```python
from build123d import *

# Parameters (mm, degrees)
SKETCH1_W           = 80
SKETCH1_H           = 60
BOSS_EXTRUDE1_DEPTH = 10
BOSS_EXTRUDE2_DEPTH = 10
LPATTERN2_COUNT     = 2
LPATTERN2_PITCH     = 70
FILLET1_R           = 5
BOSS_EXTRUDE3_START = -33.53553
BOSS_EXTRUDE3_DEPTH = 5
SKETCH4_R           = 2
CUT_EXTRUDE1_DEPTH  = 11
CUT_EXTRUDE2_DEPTH  = 81


with BuildPart() as part:
    # Sketch1 → Boss-Extrude1 (new body)
    with BuildSketch(Plane(origin=(0, 0, 0), x_dir=(1, 0, 0), z_dir=(0, 1, 0))):
        with Locations((-40, 30)):
            Rectangle(SKETCH1_W, SKETCH1_H)
    extrude(amount=BOSS_EXTRUDE1_DEPTH)

    # Sketch2 → Boss-Extrude2 (add)
    with BuildSketch(Plane(origin=(0, 0, 0), x_dir=(0, 0, -1), z_dir=(1, 0, 0))):
        Polygon((0, 10), (30, 40), (60, 10), align=None)
    boss_extrude2 = extrude(amount=-BOSS_EXTRUDE2_DEPTH)

    # LPattern2: Boss-Extrude2 ×2
    with Locations(*[(-i * LPATTERN2_PITCH, 0, 0) for i in range(1, LPATTERN2_COUNT)]):
        add(boss_extrude2)

    # Fillet1
    fillet1_edges = [part.edges().sort_by_distance(p)[0] for p in [
        (-5, 40, -30),
        (-75, 40, -30),
    ]]
    fillet(fillet1_edges, radius=FILLET1_R)

    # Sketch3 → Boss-Extrude3 (add, symmetric)
    with BuildSketch(Plane.XY.offset(BOSS_EXTRUDE3_START)):
        with BuildLine():
            Line((-70, 30), (-70, 10))
            Line((-70, 10), (-10, 10))
            Line((-10, 10), (-10, 30))
            ThreePointArc((-10, 30), (-40, 16.457513111), (-70, 30))
        make_face()
    extrude(amount=BOSS_EXTRUDE3_DEPTH, both=True)

    # Sketch4 → Cut-Extrude1 (cut, through all)
    with BuildSketch(Plane(origin=(0, 10, 0), x_dir=(1, 0, 0), z_dir=(0, 1, 0))):
        with Locations((-40, 15)):
            Circle(SKETCH4_R)
        with Locations((-35, 10)):
            Circle(SKETCH4_R)
        with Locations((-40, 5)):
            Circle(SKETCH4_R)
        with Locations((-45, 10)):
            Circle(SKETCH4_R)
    extrude(amount=-CUT_EXTRUDE1_DEPTH, mode=Mode.SUBTRACT)

    # Sketch5 → Cut-Extrude2 (cut, through all)
    with BuildSketch(Plane(origin=(0, 0, 0), x_dir=(0, 0, -1), z_dir=(1, 0, 0))):
        Polygon((43.184207347, 11.448981874), (45.338844925, 14.81907637), (43.497576267, 18.370094496), (39.501670032, 18.551018126), (37.347032454, 15.18092363), (39.188301112, 11.629905504), align=None)
    extrude(amount=-CUT_EXTRUDE2_DEPTH, mode=Mode.SUBTRACT)


solid = part.part
```
CAD build for the part. Positions are in the model's coordinates, mm. A direction names the side the tool comes from. Round coordinates to 2 decimals unless told otherwise and drop trailing zeros. Loops run counter-clockwise (first coordinate to the right, second up) from the corner with the lowest first, then second, coordinate; pieces in that order, holes last. Notation, with made-up numbers: M 2,88.25 L 25,88.25 A19 ccw 25,99.25 Z; hole C 43,58 d6. An arc over 180 degrees is marked long. Use a Markdown table: item, result. Add a question column.
(1) Drill centre lines: line 1 (X direction, y = 4.75, z = -10); line 2 (Z direction, x = -40, y = 4.75); line 3 (Z direction, x = -35, y = 6.25). Where is each one in solid material? Low to high.
(2) Cut at D-D (x = -51). Give the cut face in (y, z).
(3) Cut at B-B (x = -35). Give the cut face in (y, z).
(4) Cut at A-A (z = -15). Give the cut face in (x, y), and give its area (3 significant figures).
(5) Cut at C-C (y = 29). Give the cut face in (x, z), and give its area (3 significant figures).
(6) Flat gauge pins, fed straight in: pin 1 (6.5 mm diameter, centred on x = -56.5, y = 21, fed in from -Z); pin 2 (3 mm diameter, centred on x = -40, z = -15, fed in from -Y); pin 3 (10.5 mm diameter, centred on x = -42.5, z = -53.5, fed in from +Y); pin 4 (2 mm diameter, centred on x = -55, z = -38.5, fed in from +Y). Where does each tip first touch, or does it go through?
(7) Which spindle directions (+Z, -Z, +X, -X, +Y, -Y) get a long thin tool onto all of the face, cutting with end or side? Do faces 1 (the face through (-39.44, 16.14, -37.96)), 2 (the face through (-70, 20, -28)), 3 (the face through (-17, 21, -38.536)). Say none if no direction does.
(8) Pull direction Z, two halves, no side cores. Call faces 4 (the face through (-5.07, 37.93, -29.95)), 5 (the face through (-4.93, 16.57, -44.43)), 6 (the face through (-64, 21, -38.536)): +Z half, -Z half, draft (parallel to the pull), parting line (faces both ways), or undercut.
Geometry says:
| question | item | result |
|---|---|---|
| 1 | line 1 | x = -80 to -47, -43 to -37, -33 to 0 |
| 1 | line 2 | z = -60 to -17, -13 to -7, -3 to 0 |
| 1 | line 3 | z = -60 to -12, -8 to 0 |
| 2 | outline | M 0,-60 L 10,-60 L 10,-38.54 L 12.89,-38.54 L 15.18,-37.35 L 17.04,-38.54 L 18,-38.54 L 18,-28.54 L 10,-28.54 L 10,0 L 0,0 Z |
| 3 | outline | M 0,-60 L 10,-60 L 10,-38.54 L 12.89,-38.54 L 15.18,-37.35 L 16.77,-38.36 L 16.77,-28.54 L 10,-28.54 L 10,-12 L 0,-12 Z; M 0,-8 L 10,-8 L 10,0 L 0,0 Z |
| 4 | outline | M -80,0 L -42,0 L -42,10 L -70,10 L -70,25 L -80,25 Z; M -38,0 L 0,0 L 0,25 L -10,25 L -10,10 L -38,10 Z |
| 4 | area | 1,060 mm² |
| 5 | outline | M -80,-41 L -70,-41 L -70,-38.54 L -69.09,-38.54 L -69.09,-28.54 L -70,-28.54 L -70,-19 L -80,-19 Z; M -10.91,-38.54 L -10,-38.54 L -10,-41 L 0,-41 L 0,-19 L -10,-19 L -10,-28.54 L -10.91,-28.54 Z |
| 5 | area | 458 mm² |
| 6 | pin 1 | stops at z = -38.54 |
| 6 | pin 2 | passes through |
| 6 | pin 3 | stops at y = 10 |
| 6 | pin 4 | stops at y = 19.8 |
| 7 | face 1 | +X, -X |
| 7 | face 2 | +Y |
| 7 | face 3 | -Z, +Y |
| 8 | face 4 | parting line |
| 8 | face 5 | undercut |
| 8 | face 6 | -Z half |
